```python
from build123d import *

# Parameters (mm, degrees)
CROQUIS1_W              = 350
CROQUIS1_H              = 80
CROQUIS1_R              = 30
CROQUIS1_R_2            = 10
SALIENTE_EXTRUIR1_DEPTH = 15


with BuildPart() as part:
    # Croquis1 → Saliente-Extruir1 (new body)
    with BuildSketch(Plane.XY):
        Rectangle(CROQUIS1_W, CROQUIS1_H)
        Circle(CROQUIS1_R, mode=Mode.SUBTRACT)
        with Locations((150, 0)):
            Circle(CROQUIS1_R_2, mode=Mode.SUBTRACT)
        with Locations((-150, 0)):
            Circle(CROQUIS1_R_2, mode=Mode.SUBTRACT)
    extrude(amount=-SALIENTE_EXTRUIR1_DEPTH)


solid = part.part
```
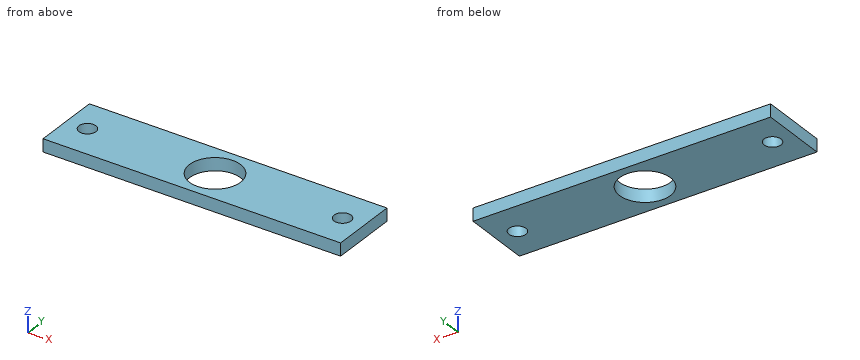
Verification items for the finished model (mm, model axes). Coordinates: 2 decimals unless noted, no trailing zeros. Loops run counter-clockwise (first coordinate to the right, second up) from the corner with the lowest first, then second, coordinate; pieces in that order, holes last. Notation, with made-up numbers: (-36, -24.75) -> (14, -24.75) arc R30 cw to (14, -2.75) -> close; hole circle Ø3 at (-39, 65.5). An arc over 180 degrees is marked (long way). Put each result on its own line as item: value.
1. Section check D-D, the plane x = 0. Record the boundary of the cut face in (y, z).
Result set:
outline: (-40, -15) -> (-30, -15) -> (-30, 0) -> (-40, 0) -> close; (30, -15) -> (40, -15) -> (40, 0) -> (30, 0) -> close
2. Section check C-C, the plane y = 4. Record the boundary of the cut face in (x, z).
Result set:
outline: (-175, -15) -> (-159.17, -15) -> (-159.17, 0) -> (-175, 0) -> close; (-140.83, -15) -> (-29.73, -15) -> (-29.73, 0) -> (-140.83, 0) -> close; (29.73, -15) -> (140.83, -15) -> (140.83, 0) -> (29.73, 0) -> close; (159.17, -15) -> (175, -15) -> (175, 0) -> (159.17, 0) -> close
3. Section check A-A, the plane x = 150. Record the boundary of the cut face in (y, z), then the cut area to 3 significant figures.
Result set:
outline: (-40, -15) -> (-10, -15) -> (-10, 0) -> (-40, 0) -> close; (10, -15) -> (40, -15) -> (40, 0) -> (10, 0) -> close
area: 900 mm^2
4. Section check B-B, the plane z = -4.75. Record the boundary of the cut face in (x, y), then the cut area to 3 significant figures.
Result set:
outline: (-175, -40) -> (175, -40) -> (175, 40) -> (-175, 40) -> close; hole circle Ø20 at (-150, 0); hole circle Ø60 at (0, 0); hole circle Ø20 at (150, 0)
area: 24,500 mm^2
5. Thickness scan on line 1 (X direction, y = 1, z = -11.75); line 2 (X direction, y = 4, z = -5.5); line 3 (Y direction, x = -150, z = -7.25). Record the ranges inside material, lowest first.
Result set:
line 1: x = -175 to -159.95, -140.05 to -29.98, 29.98 to 140.05, 159.95 to 175
line 2: x = -175 to -159.17, -140.83 to -29.73, 29.73 to 140.83, 159.17 to 175
line 3: y = -40 to -10, 10 to 40
